Verification items for this drawing (mm, ordinates from the low corner). A direction names the side the tool comes from. Round coordinates to 2 decimals unless told otherwise and drop trailing zeros. Loops run counter-clockwise (first coordinate to the right, second up) from the corner with the lowest first, then second, coordinate; pieces in that order, holes last. Notation, with made-up numbers: M -26,39 L -11,39 A13 cw -11,51 Z; hole C -9,68 d6. An arc over 180 degrees is marked long. Write item = value, one per line.
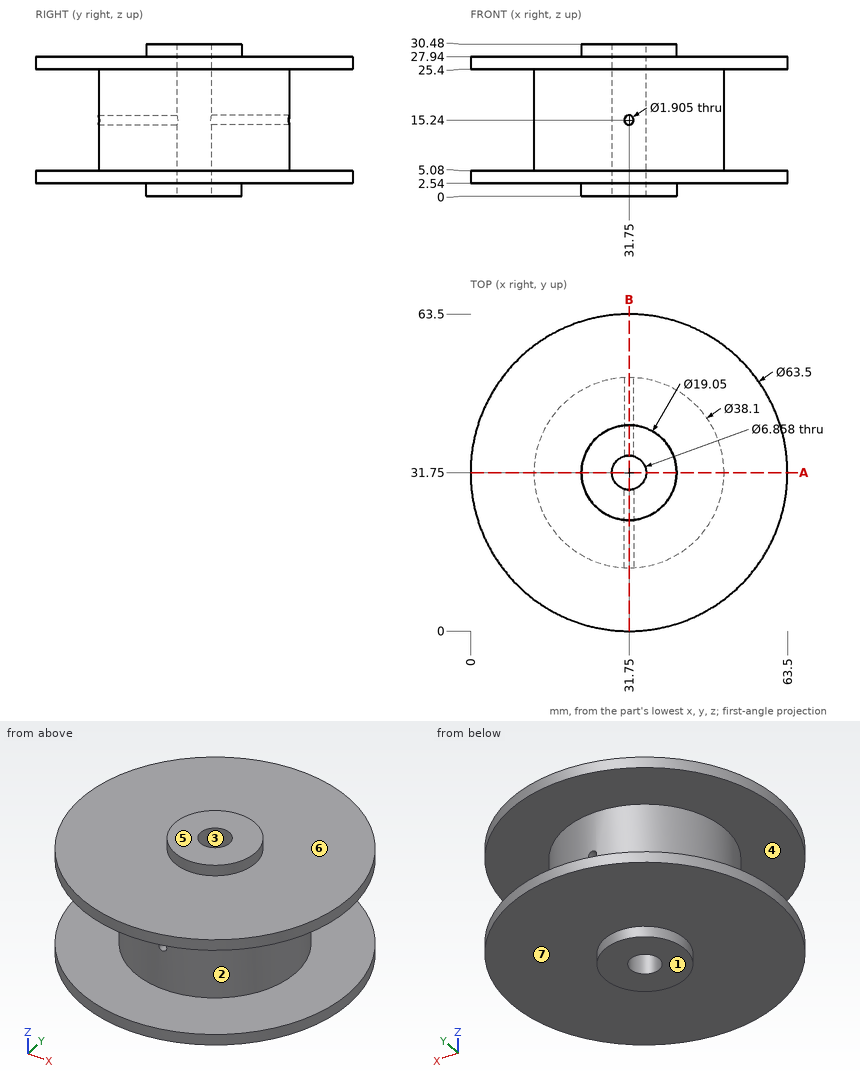
(1) Release check for a two-part mould opening along X. For the marked faces 1, 2 and 3 record: released by +X, released by -X, zero draft, split by the parting line, or undercut.
Result set:
face_1 = zero draft
face_2 = split by the parting line
face_3 = undercut
(2) Material ranges on line 1 along Z through (x, y) = (43, 51); line 2 along Y through (x, z) = (32, 25); line 3 along Z through (x, y) = (31.75, 46.5), recorded low to high. Write a range as from..to.
Result set:
line_1 = 2.54..5.08, 25.4..27.94
line_2 = 12.7..28.33, 35.17..50.8
line_3 = 2.54..14.29, 16.19..27.94
(3) Depth check by flat-ended pin: pin 1 Ø10 at (x, y) = (50, 49) entering from -Z; pin 2 Ø6 at (x, z) = (35, 5.5) entering from +Y; pin 3 Ø3 at (x, z) = (31.75, 15.24) entering from -Y. Enter the tip coordinate at first touch or a pass-through.
Result set:
pin_1 = 2.54
pin_2 = 63.5
pin_3 = 12.7
(4) Sectioned sample at A-A on y = 31.75. Record the cut outline in (x, z) (3 decimals), then the cut area to 3 significant figures.
Result set:
outline = M 0,2.54 L 22.225,2.54 L 22.225,0 L 28.321,0 L 28.321,30.48 L 22.225,30.48 L 22.225,27.94 L 0,27.94 L 0,25.4 L 12.7,25.4 L 12.7,5.08 L 0,5.08 Z; M 35.179,0 L 41.275,0 L 41.275,2.54 L 63.5,2.54 L 63.5,5.08 L 50.8,5.08 L 50.8,25.4 L 63.5,25.4 L 63.5,27.94 L 41.275,27.94 L 41.275,30.48 L 35.179,30.48 Z
area = 985 mm2
(5) Sectioned sample at B-B on x = 31.75. State how many separate pieces and enclosed holes the cut face has, then the cut area to 3 significant figures.
Result set:
separate_pieces = 4
enclosed_holes = 0
area = 925 mm2
(6) Tool access check on the marked faces 4, 5, 6 and 7. Record the directions out of +Z, -Z, +X, -X, +Y, -Y that give a thin tool (end or side, any length) a straight path to the whole face; none if there is none.
Result set:
face_4 = none
face_5 = +Z, +X, -X, +Y, -Y
face_6 = +Z
face_7 = -Z
